from build123d import *

# Parameters (mm, degrees)
F0_R     = 7
F1_DEPTH = 28.8
F2_DEPTH = 10
F3_DEPTH = 10
F4_W     = 27.706493
F4_H     = 12
F4_R     = 3.4
F5_DEPTH = 29.9


with BuildPart() as f1:
    # F0 (on Front) → F1 (new body)
    with BuildSketch(Plane.XZ):
        with BuildLine():
            ThreePointArc((-40.688801, 13.714286), (-61.636868, 19.855844), (-52.56572, 0))
            Line((-52.56572, 0), (-5.20572, 0))
            Line((-5.20572, 0), (-10.20572, 12))
            Line((-10.20572, 12), (-38.709314, 12))
            ThreePointArc((-38.709314, 12), (-40.018621, 12.488142), (-40.688801, 13.714286))
        make_face()
        with Locations((-52.56572, 12)):
            Circle(F0_R, mode=Mode.SUBTRACT)
        with BuildLine():
            Line((4.79428, 12), (4.79428, 0))
            Line((4.79428, 0), (47.43428, 0))
            Line((47.43428, 0), (47.43428, 8))
            ThreePointArc((47.43428, 8), (46.262707, 10.828427), (43.43428, 12))
            Line((43.43428, 12), (24.43428, 12))
            Line((24.43428, 12), (4.79428, 12))
        make_face()
        Polygon((-10.20572, 12), (-5.20572, 0), (4.79428, 0), (4.79428, 12), align=None)
    extrude(amount=-F1_DEPTH)

    # F0 (on Front) → F2 (join)
    with BuildSketch(Plane.XZ):
        with BuildLine():
            ThreePointArc((12.43428, 32), (10.459133, 21.295266), (4.79428, 12))
            Line((4.79428, 12), (24.43428, 12))
            ThreePointArc((24.43428, 12), (23.020066, 12.585786), (22.43428, 14))
            Line((22.43428, 14), (22.43428, 28))
            ThreePointArc((22.43428, 28), (21.262707, 30.828427), (18.43428, 32))
            Line((18.43428, 32), (12.43428, 32))
        make_face()
    extrude(amount=-F2_DEPTH)

    # F0 (on Front) → F3 (cut)
    with BuildSketch(Plane.XZ):
        Polygon((-10.20572, 12), (-5.20572, 0), (4.79428, 0), (4.79428, 12), align=None)
    extrude(amount=-F3_DEPTH, mode=Mode.SUBTRACT)

    # F4 (on Top) → F5 (cut)
    with BuildSketch(Plane.XY):
        with Locations((-50.712474, 14.4)):
            Rectangle(F4_W, F4_H)
        with Locations((20.43428, 19.4)):
            Circle(F4_R)
    extrude(amount=F5_DEPTH, mode=Mode.SUBTRACT)


solid = f1.part
Geometry: final body of the model. Coordinates: model frame, mm. A direction names the side the tool comes from. Give positions to 0.01 mm unless a question says otherwise; leave off trailing zeros. Write each loop counter-clockwise with the first axis right and the second up, starting at its lowest first coordinate (ties: lowest second). Pieces come first, ordered by that corner, then holes. Notation, with made-up numbers: (60, 35) -> (73, 35) arc R32 ccw to (73, 69) -> close; hole circle Ø7 at (68, 63.5). An arc over 180 degrees is marked (long way). Answer in a Markdown table with one row per item.
(1) Section query C-C on z = 21. Return loops of the section in (x, y), then the cut area to 3 significant figures.
Answers below:
| item | result |
|---|---|
| outline | (-60.5, 0) -> (-44.63, 0) -> (-44.63, 8.4) -> (-60.5, 8.4) -> close; (-60.5, 20.4) -> (-44.63, 20.4) -> (-44.63, 28.8) -> (-60.5, 28.8) -> close; (10.34, 0) -> (22.43, 0) -> (22.43, 10) -> (10.34, 10) -> close |
| area | 388 mm^2 |
(2) Section query A-A on y = 19.4. Return loops of the section in (x, z).
Answers below:
| item | result |
|---|---|
| outline | (-36.86, 0) -> (17.03, 0) -> (17.03, 12) -> (-36.86, 12) -> close; (23.83, 0) -> (47.43, 0) -> (47.43, 8) arc R4 ccw to (43.43, 12) -> (23.83, 12) -> close |
(3) Pin query (flat end, axial travel): pin 1 (3 mm diameter, centred on x = 22.5, z = 27.5, fed in from +Y); pin 2 (3 mm diameter, centred on y = 12, z = 19.5, fed in from +X); pin 3 (13 mm diameter, centred on y = 15, z = 7.5, fed in from -X); pin 4 (8 mm diameter, centred on y = 6.5, z = 23, fed in from +X). Return the tip coordinate at first contact, or that it passes through.
Answers below:
| item | result |
|---|---|
| pin 1 | y = 10 |
| pin 2 | through |
| pin 3 | x = -64.53 |
| pin 4 | x = 22.43 |
(4) Draft query along X for faces 1 (the cylindrical face through (-61.381, 24.541, 20.142)), 2 (the cylindrical face through (10.5, 4.9, 21.4)), 3 (the flat face through (-48, 8.4, 6)), 4 (the flat face through (4.794, 5, 6)). Return one class per face: +X half, -X half, draft (parallel to the pull), parting line (faces both ways), or undercut.
Answers below:
| item | result |
|---|---|
| face 1 | parting line |
| face 2 | undercut |
| face 3 | draft |
| face 4 | undercut |
(5) Ray query, line 1 along X through (y, z) = (5, 14.5); line 2 along Z through (x, y) = (-52.5, 6.25); line 3 along Y through (x, z) = (22, 15.5). Return the intervals inside material, ascending. Write a range as [from, to].
Answers below:
| item | result |
|---|---|
| line 1 | [-64.3, -59.1], [-46.03, -40.83], [6.8, 22.43] |
| line 2 | [0, 5], [19, 24] |
| line 3 | [0, 10] |
(6) Section query B-B on z = 6.5. Return loops of the section in (x, y), then the cut area to 3 significant figures.
Answers below:
| item | result |
|---|---|
| outline | (-63.23, 0) -> (-56.9, 0) -> (-56.9, 8.4) -> (-63.23, 8.4) -> close; (-63.23, 20.4) -> (-56.9, 20.4) -> (-56.9, 28.8) -> (-63.23, 28.8) -> close; (-48.24, 0) -> (-7.91, 0) -> (-7.91, 10) -> (4.79, 10) -> (4.79, 0) -> (47.43, 0) -> (47.43, 28.8) -> (-48.24, 28.8) -> (-48.24, 20.4) -> (-36.86, 20.4) -> (-36.86, 8.4) -> (-48.24, 8.4) -> close; hole circle Ø6.8 at (20.43, 19.4) |
| area | 2,560 mm^2 |
(7) Set-up query: faces 5 (the cylindrical face through (17.038, 19.549, 5.916)), 6 (the flat face through (-36.859, 14, 6)), 7 (the flat face through (-1, 10, 6)). Return all of +Z, -Z, +X, -X, +Y, -Y with unobstructed straight access to the full face (end or side cutting, diameter ignored); none if empty.
Answers below:
| item | result |
|---|---|
| face 5 | +Z, -Z |
| face 6 | +Z, -Z, -X |
| face 7 | +Z, -Y |
(8) Section query D-D on x = -20. Return loops of the section in (y, z).
Answers below:
| item | result |
|---|---|
| outline | (0, 0) -> (28.8, 0) -> (28.8, 12) -> (0, 12) -> close |
